Source: CAD feature listing. Evaluate the final solid. Frame: model axes, mm. A direction names the side the tool comes from. Give positions to 0.01 mm unless a question says otherwise; leave off trailing zeros. Loops run counter-clockwise (first coordinate to the right, second up) from the corner with the lowest first, then second, coordinate; pieces in that order, holes last. Notation, with made-up numbers: M 39.5,48.5 L 72.5,48.5 A11 cw 72.5,63.5 Z; hole C 63.25,-19 d3. An arc over 180 degrees is marked long. Answer in a Markdown table with one row per item.
```python
from build123d import *

# Parameters (mm, degrees)
MODEL_R                     = 2.5
DODANIE_WYCI_GNI_CIE1_DEPTH = 10


with BuildPart() as part:
    # Model → Dodanie-wyciągnięcie1 (new body)
    with BuildSketch(Plane.XY):
        Polygon((229.573669216, 20), (20.573669216, 24), (0.073669216, 24), (0.073669216, -3.757619404), (20.573669216, -3.757619404), (229.573669216, 0), (250.073669216, 0), (250.073669216, 20), align=None)
        with Locations((10.073669216, 17.121190298)):
            Circle(MODEL_R, mode=Mode.SUBTRACT)
        with Locations((240.073669216, 10)):
            Circle(MODEL_R, mode=Mode.SUBTRACT)
        with Locations((10.073669216, 2.878809702)):
            Circle(MODEL_R, mode=Mode.SUBTRACT)
        with Locations((125.073669216, 10)):
            Circle(MODEL_R, mode=Mode.SUBTRACT)
        with BuildLine():
            Line((215.057391591, 13.621190298), (143.897703929, 15.259018411))
            ThreePointArc((143.897703929, 15.259018411), (138.390896743, 10), (143.897703929, 4.740981589))
            Line((143.897703929, 4.740981589), (215.057391591, 6.378809702))
            ThreePointArc((215.057391591, 6.378809702), (218.678581889, 10), (215.057391591, 13.621190298))
        make_face(mode=Mode.SUBTRACT)
        with BuildLine():
            Line((106.398152108, 15.914510504), (38.806300427, 17.270637985))
            ThreePointArc((38.806300427, 17.270637985), (31.237940567, 10), (38.806300427, 2.729362015))
            Line((38.806300427, 2.729362015), (106.398152108, 4.085489496))
            ThreePointArc((106.398152108, 4.085489496), (112.312662612, 10), (106.398152108, 15.914510504))
        make_face(mode=Mode.SUBTRACT)
    extrude(amount=DODANIE_WYCI_GNI_CIE1_DEPTH)


solid = part.part
```
Q1. Ray query, probe 1 along X at (y, z) = (8.75, 5.5); probe 2 along X at (y, z) = (0.75, 4.75); probe 3 along Y at (x, z) = (111.5, 2.75). Return the intervals inside material, ascending. Write a range as from..to.
Values follow:
| item | result |
|---|---|
| probe 1 | 0.07..31.35, 112.18..122.91, 127.24..138.54, 218.46..237.91, 242.24..250.07 |
| probe 2 | 0.07..8.76, 11.38..250.07 |
| probe 3 | -2.12..7.01, 12.99..22.26 |
Q2. Contact query for flat-ended pins moving along their axis: pin 1 Ø5 at (x, z) = (123.5, 3.5) entering from +Y; pin 2 Ø5 at (x, z) = (238, 2.5) entering from -Y; pin 3 Ø3 at (x, z) = (44, 6.5) entering from -Y. Output: stop coordinate, or through.
Values follow:
| item | result |
|---|---|
| pin 1 | y = 22.08 |
| pin 2 | y = 0 |
| pin 3 | y = -3.36 |
Q3. Mould query, pull axis X, two halves, no side actions, for faces 4 (the flat face through (0.074, 10, 5)), 5 (the flat face through (123, 7, 10)), 6 (the cylindrical face through (242.38, 9.04, 4.93)), 7 (the flat face through (250.074, 10, 5)). Classes: +X half, -X half, draft (parallel to the pull), parting line (faces both ways), or undercut.
Values follow:
| item | result |
|---|---|
| face 4 | -X half |
| face 5 | draft |
| face 6 | undercut |
| face 7 | +X half |
Q4. Reachability of faces 1 (the flat face through (240, 0, 5)), 2 (the flat face through (10, 24, 5)), 3 (the cylindrical face through (112.31, 9.87, 4.93)) from +Z, -Z, +X, -X, +Y, -Y: full face, straight path, thin tool, end or side. Return the list, or none.
Values follow:
| item | result |
|---|---|
| face 1 | +Z, -Z, +X, -Y |
| face 2 | +Z, -Z, +X, -X, +Y |
| face 3 | +Z, -Z |
Q5. Section query B-B (z = 2.25). Output: boundary loops of the cut face in (x, y), plus the area to 3 significant figures.
Values follow:
| item | result |
|---|---|
| outline | M 0.07,-3.76 L 20.57,-3.76 L 229.57,0 L 250.07,0 L 250.07,20 L 229.57,20 L 20.57,24 L 0.07,24 Z; hole C 10.07,2.88 d5; hole C 10.07,17.12 d5; hole M 38.81,2.73 L 106.4,4.09 A5.91 ccw 106.4,15.91 L 38.81,17.27 A7.28 ccw long Z; hole C 125.07,10 d5; hole M 143.9,4.74 L 215.06,6.38 A3.62 ccw 215.06,13.62 L 143.9,15.26 A5.26 ccw long Z; hole C 240.07,10 d5 |
| area | 4,160 mm^2 |
Q6. Section query A-A (y = 10). Output: boundary loops of the cut face in (x, z), plus the area to 3 significant figures.
Values follow:
| item | result |
|---|---|
| outline | M 0.07,0 L 31.24,0 L 31.24,10 L 0.07,10 Z; M 112.31,0 L 122.57,0 L 122.57,10 L 112.31,10 Z; M 127.57,0 L 138.39,0 L 138.39,10 L 127.57,10 Z; M 218.68,0 L 237.57,0 L 237.57,10 L 218.68,10 Z; M 242.57,0 L 250.07,0 L 250.07,10 L 242.57,10 Z |
| area | 786 mm^2 |
